Model file for the job. Use its own axes, mm. Give positions to 0.01 mm unless a question says otherwise; leave off trailing zeros. Order: outer loops, then holes, each group sorted by start corner. A loop starts at its lowest first (then second) coordinate and runs counter-clockwise, first axis right, second up. Notation, with made-up numbers: (-12, 73) -> (31, 73) arc R12 ccw to (31, 96) -> close; hole circle Ø2 at (60.5, 48.25). An arc over 180 degrees is marked (long way). Use CSV: the item, a comma, the result in double quotes. Start each with the question number.
1. Cut at B-B on y = 0.85. List the corners of the cut face in (x, z) (1 decimal).
2. Cut at D-D on x = 11. List the corners of the cut face in (y, z).
3. Wall check: line 1 (X direction, y = 1.5, z = 0); line 2 (X direction, y = 4, z = 0); line 3 (Z direction, x = 56.5, y = 1.4). Give the ranges that are in metal, low to high. Write a range as from..to.
4. Cut at A-A on x = 74.5. List the corners of the cut face in (y, z), then the cut area to 3 significant figures.
5. Drop flat-ended pins along their axis: pin 1 (8 mm diameter, centred on x = 15, z = -7.5, fed in from -Y); pin 2 (2.5 mm diameter, centred on x = 0, z = 0, fed in from +Y) (3 decimals); pin 3 (2 mm diameter, centred on x = 62.5, y = 2.5, fed in from -Z); pin 4 (2.5 mm diameter, centred on x = 101, z = 1.5, fed in from -Y). Give the stop position or say it passes through.
6. Cut at C-C on z = 7. List the corners of the cut face in (x, y).
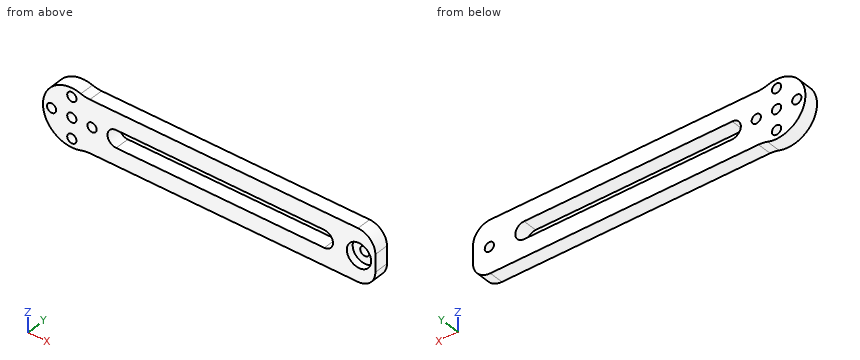
```python
from build123d import *

# Parameters (mm, degrees)
SKETCH_1_R          = 1.6
SKETCH_1_R_2        = 9
EXTRUDE_1_DEPTH     = 5
SKETCH_2_R          = 4.2
CUT_EXTRUDE_1_DEPTH = 2.5
EXTRUDE_START       = -5
SKETCH_3_R          = 10
SKETCH_3_R_2        = 9
EXTRUDE_2_DEPTH     = 5
FILLET_1_R          = 10


with BuildPart() as part:
    # 草图1 → 凸台-拉伸1 (new body)
    # profile 1 of 2: a face of its own
    with BuildSketch(Plane(origin=(0, 0, 0), x_dir=(1, 0, 0), z_dir=(0, 1, 0))):
        with BuildLine():
            Line((99, 9), (0, 9))
            ThreePointArc((0, 9), (6.363961031, 6.363961031), (9, 0))
            ThreePointArc((9, 0), (6.363961031, -6.363961031), (0, -9))
            Line((0, -9), (99, -9))
            ThreePointArc((99, -9), (103.242640687, -7.242640687), (105, -3))
            Line((105, -3), (105, 3))
            ThreePointArc((105, 3), (103.242640687, 7.242640687), (99, 9))
        make_face()
        with BuildLine():
            ThreePointArc((15.34, -3), (12.34, 0), (15.34, 3))
            Line((15.34, 3), (87.34, 3))
            ThreePointArc((87.34, 3), (90.34, 0), (87.34, -3))
            Line((87.34, -3), (15.34, -3))
        make_face(mode=Mode.SUBTRACT)
        with Locations(Location((99.34, 0, 0), (0, 0, 270))):
            Circle(SKETCH_1_R, mode=Mode.SUBTRACT)
    # profile 2 of 2: a face of its own
    with BuildSketch(Plane(origin=(0, 0, 0), x_dir=(1, 0, 0), z_dir=(0, 1, 0))):
        Circle(SKETCH_1_R_2)
        with Locations(Location((0, -7, 0), (0, 0, 270))):
            Circle(SKETCH_1_R, mode=Mode.SUBTRACT)
        with Locations(Location((7, 0, 0), (0, 0, 270))):
            Circle(SKETCH_1_R, mode=Mode.SUBTRACT)
        with Locations(Location((0, 7, 0), (0, 0, 270))):
            Circle(SKETCH_1_R, mode=Mode.SUBTRACT)
        with Locations(Location((-7, 0, 0), (0, 0, 270))):
            Circle(SKETCH_1_R, mode=Mode.SUBTRACT)
        with Locations(Location((0, 0, 0), (0, 0, 270))):
            Circle(SKETCH_1_R, mode=Mode.SUBTRACT)
    extrude(amount=EXTRUDE_1_DEPTH)

    # 草图2 → 切除-拉伸1 (cut)
    with BuildSketch(Plane.XZ):
        with Locations(Location((99.34, 0, 0), (0, 0, 270))):
            Circle(SKETCH_2_R)
    extrude(amount=-CUT_EXTRUDE_1_DEPTH, mode=Mode.SUBTRACT)

    # 草图3 → 凸台-拉伸2 (add)
    with BuildSketch(Plane(origin=(0, 5, 0), x_dir=(1, 0, 0), z_dir=(0, 1, 0)).offset(EXTRUDE_START)):
        Circle(SKETCH_3_R)
        Circle(SKETCH_3_R_2, mode=Mode.SUBTRACT)
    extrude(amount=EXTRUDE_2_DEPTH)

    # 圆角1
    fillet_1_edges = [part.edges().sort_by_distance(p)[0] for p in [
        (4.358898944, 2.5, -9),
        (4.358898944, 2.5, 9),
    ]]
    fillet(fillet_1_edges, radius=FILLET_1_R)


solid = part.part
```
Verdict:
1,outline,"(3.1, -9.5) arc R10 cw to (6.2, -9) -> (99, -9) arc R6 ccw to (105, -3) -> (105, 3) arc R6 ccw to (99, 9) -> (6.2, 9) arc R10 cw to (3.1, 9.5) arc R10 ccw (long way) to start; hole circle Ø3.2 at (-7, 0); hole circle Ø3.2 at (0, -7); hole circle Ø3.2 at (0, 0); hole circle Ø3.2 at (0, 7); hole circle Ø3.2 at (7, 0); hole (15.3, -3) -> (87.3, -3) arc R3 ccw to (87.3, 3) -> (15.3, 3) arc R3 ccw to start; hole circle Ø8.4 at (99.3, 0)"
2,outline,"(0, -9) -> (5, -9) -> (5, 9) -> (0, 9) -> close"
3,line 1,"-10..-8.6, -5.4..-1.6, 1.6..5.4, 8.6..12.34, 90.34..95.14, 103.54..105"
3,line 2,"-10..-8.6, -5.4..-1.6, 1.6..5.4, 8.6..12.34, 90.34..97.74, 100.94..105"
3,line 3,"-9..-3, 3..9"
4,outline,"(0, -9) -> (5, -9) -> (5, -3) -> (0, -3) -> close; (0, 3) -> (5, 3) -> (5, 9) -> (0, 9) -> close"
4,area,"60.0 mm^2"
5,pin 1,"y = 0"
5,pin 2,"through"
5,pin 3,"z = -9"
5,pin 4,"y = 2.5"
6,outline,"(-7.14, 0) -> (-1.6, 0) -> (-1.6, 5) -> (-7.14, 5) -> close; (1.6, 0) -> (103.47, 0) -> (103.47, 5) -> (1.6, 5) -> close"
